from build123d import *

# Parameters (mm, degrees)
F0_R           = 5.5
F0_R_2         = 2
F1_DEPTH       = 43
F3_SIZE        = 0.15
F2_R           = 2.25
F2_R_2         = 2
F5_DEPTH       = 2
F6_R           = 5
F8_D           = 4
F8_DEPTH       = 1.5
F8_TIP         = 1.2017212381
F8_ON_F4_D     = 4
F8_ON_F4_DEPTH = 1.5
F8_ON_F4_TIP   = 1.2017212381


with BuildPart() as f1:
    # F0 (on Top) → F1 (new body)
    with BuildSketch(Plane.XY):
        with BuildLine():
            ThreePointArc((0, 6), (-6, 12), (-12, 6))
            ThreePointArc((-12, 6), (-18, 12), (-24, 6))
            Line((-24, 6), (-24, -6))
            ThreePointArc((-24, -6), (-18, -12), (-12, -6))
            ThreePointArc((-12, -6), (-6, -12), (0, -6))
            ThreePointArc((0, -6), (6, -12), (12, -6))
            ThreePointArc((12, -6), (18, -12), (24, -6))
            Line((24, -6), (24, 6))
            ThreePointArc((24, 6), (18, 12), (12, 6))
            ThreePointArc((12, 6), (6, 12), (0, 6))
        make_face()
        with Locations((-18, -6)):
            Circle(F0_R, mode=Mode.SUBTRACT)
        with Locations((-6, -6)):
            Circle(F0_R, mode=Mode.SUBTRACT)
        with Locations((6, -6)):
            Circle(F0_R, mode=Mode.SUBTRACT)
        with Locations((18, -6)):
            Circle(F0_R, mode=Mode.SUBTRACT)
        with Locations((-12, 0)):
            Circle(F0_R_2, mode=Mode.SUBTRACT)
        with Locations((-18, 6)):
            Circle(F0_R, mode=Mode.SUBTRACT)
        with Locations((-6, 6)):
            Circle(F0_R, mode=Mode.SUBTRACT)
        Circle(F0_R_2, mode=Mode.SUBTRACT)
        with Locations((12, 0)):
            Circle(F0_R_2, mode=Mode.SUBTRACT)
        with Locations((6, 6)):
            Circle(F0_R, mode=Mode.SUBTRACT)
        with Locations((18, 6)):
            Circle(F0_R, mode=Mode.SUBTRACT)
    extrude(amount=F1_DEPTH)

    # F3
    f3_edges = [f1.edges().sort_by_distance(p)[0] for p in [
        (-23.5, 6, 43),
        (-11.5, 6, 43),
        (0.5, 6, 43),
        (12.5, 6, 43),
        (12.5, -6, 43),
        (0.5, -6, 43),
        (-11.5, -6, 43),
        (-23.5, -6, 43),
    ]]
    chamfer(f3_edges, length=F3_SIZE)

    # F2 (on face) → F5 (join)
    with BuildSketch(Plane(origin=(0, 0, 0), x_dir=(1, 0, 0), z_dir=(0, 0, -1))):
        with BuildLine():
            ThreePointArc((12, 6), (6, 12), (0, 6))
            ThreePointArc((0, 6), (-6, 12), (-12, 6))
            ThreePointArc((-12, 6), (-18, 12), (-24, 6))
            Line((-24, 6), (-24, -6))
            ThreePointArc((-24, -6), (-18, -12), (-12, -6))
            ThreePointArc((-12, -6), (-6, -12), (0, -6))
            ThreePointArc((0, -6), (6, -12), (12, -6))
            ThreePointArc((12, -6), (18, -12), (24, -6))
            Line((24, -6), (24, 6))
            ThreePointArc((24, 6), (18, 12), (12, 6))
        make_face()
        with Locations((-18, -6)):
            Circle(F2_R, mode=Mode.SUBTRACT)
        with Locations((-6, -6)):
            Circle(F2_R, mode=Mode.SUBTRACT)
        with Locations((6, -6)):
            Circle(F2_R, mode=Mode.SUBTRACT)
        with Locations((18, -6)):
            Circle(F2_R, mode=Mode.SUBTRACT)
        with Locations((-12, 0)):
            Circle(F2_R_2, mode=Mode.SUBTRACT)
        with Locations((-18, 6)):
            Circle(F2_R, mode=Mode.SUBTRACT)
        with Locations((-6, 6)):
            Circle(F2_R, mode=Mode.SUBTRACT)
        Circle(F2_R_2, mode=Mode.SUBTRACT)
        with Locations((12, 0)):
            Circle(F2_R_2, mode=Mode.SUBTRACT)
        with Locations((6, 6)):
            Circle(F2_R, mode=Mode.SUBTRACT)
        with Locations((18, 6)):
            Circle(F2_R, mode=Mode.SUBTRACT)
    extrude(amount=F5_DEPTH)

    # F6
    f6_edges = [f1.edges().sort_by_distance(p)[0] for p in [
        (12, -6, 20.5),
        (0, -6, 20.5),
        (-12, -6, 20.5),
        (12, 6, 20.5),
        (0, 6, 20.5),
        (-12, 6, 20.5),
    ]]
    fillet(f6_edges, radius=F6_R)

    # F8
    with Locations(Plane.YZ.offset(24)):
        with Locations((0, 39)):
            Hole(F8_D / 2, depth=F8_DEPTH)
            with Locations((0, 0, -(F8_DEPTH + F8_TIP / 2))):  # 118° drill point
                Cone(0, F8_D / 2, F8_TIP, mode=Mode.SUBTRACT)

    # F8 on F4
    with Locations(Plane(origin=(-24, 0, 0), x_dir=(0, -1, 0), z_dir=(-1, 0, 0))):
        with Locations((0, 39)):
            Hole(F8_ON_F4_D / 2, depth=F8_ON_F4_DEPTH)
            with Locations((0, 0, -(F8_ON_F4_DEPTH + F8_ON_F4_TIP / 2))):  # 118° drill point
                Cone(0, F8_ON_F4_D / 2, F8_ON_F4_TIP, mode=Mode.SUBTRACT)


solid = f1.part
The listing builds one solid part. Answer for the finished solid, in the listing's coordinates (mm). A direction names the side the tool comes from. Coordinates: 2 decimals unless noted, no trailing zeros. Order: outer loops, then holes, each group sorted by start corner. A loop starts at its lowest first (then second) coordinate and runs counter-clockwise, first axis right, second up.
Q1. A cutting plane is placed at B-B, the plane y = 7.5. State how many separate pieces and enclosed holes the cut face has, and give its area (3 significant figures).
Q2. Given P1, Ø5.5, axis at x = -6.5, y = 4.5, coming from the +Z side; P2, Ø5.5, axis at x = 16, y = -4, coming from the +Z side; P3, Ø1, axis at x = -14, z = 27, coming from the -Y side, each flat-ended and moving along its own axis, determine where each tip first touches the part or whether it passes through.
Q3. For a pull along X with two mould halves and no side action, classify faces 1 (the face through (23, 0, 37)), 2 (the face through (16.81, -11.37, 21.13)), 3 (the face through (-3.6, -6.1, 0)), 4 (the face through (21.507, -0.045, 39.344)) as pulls with the +X half, pulls with the -X half, needs draft (parallel to the pull), parting line crosses it, or undercut.
Q4. Consider line 1 (X direction, y = -5.75, z = 1); line 2 (X direction, y = 0, z = 24); line 3 (Y direction, x = -18, z = 26). Determine where each line is inside the solid, lowest interval first.
Q5. Which of the six approach directions +Z, -Z, +X, -X, +Y, -Y give full straight-line access (tool end or side, diameter ignored) to faces 5 (the face through (8.4, -6.1, 0)), 6 (the face through (-20.94, 11.23, 20.82))?
Q6. A cutting plane is placed at A-A, the plane x = 18. Write down the section's boundary in (y, z), and give its area (3 significant figures).
Answers follow:
1. separate pieces: 5
1. enclosed holes: 0
1. area: 296 mm2
2. P1: stops at z = 0
2. P2: stops at z = 42.93
2. P3: stops at y = -10.89
3. face 1: needs draft
3. face 2: undercut
3. face 3: undercut
3. face 4: pulls with the +X half
4. line 1: x = -24 to -23.49, -12.51 to -11.49, -0.51 to 0.51, 11.49 to 12.51, 23.49 to 24
4. line 2: x = -24 to -14, -10 to -2, 2 to 10, 14 to 24
4. line 3: y = -12 to -11.5, -0.5 to 0.5, 11.5 to 12
5. face 5: +Z
5. face 6: +Z, -Z, +Y
6. outline: (-12, -2) - (-8.25, -2) - (-8.25, 0) - (-11.5, 0) - (-11.5, 42.85) - (-11.65, 43) - (-12, 43) - close; (-3.75, -2) - (3.75, -2) - (3.75, 0) - (0.5, 0) - (0.5, 42.85) - (0.35, 43) - (-0.35, 43) - (-0.5, 42.85) - (-0.5, 0) - (-3.75, 0) - close; (8.25, -2) - (12, -2) - (12, 43) - (11.65, 43) - (11.5, 42.85) - (11.5, 0) - (8.25, 0) - close
6. area: 116 mm2
